Build history of the part. All positions in model axes, mm. A direction names the side the tool comes from. Round coordinates to 2 decimals unless told otherwise and drop trailing zeros. Write each loop counter-clockwise with the first axis right and the second up, starting at its lowest first coordinate (ties: lowest second). Pieces come first, ordered by that corner, then holes. Notation, with made-up numbers: M 82.25,64.25 L 93.25,64.25 A21 ccw 93.25,76.25 Z; hole C -37.5,5.5 d1. An arc over 180 degrees is marked long. Use a Markdown table: item, result.
from build123d import *

# Parameters (mm, degrees)
F0_R     = 3.96875
F1_DEPTH = 6.3246


with BuildPart() as f1:
    # F0 (on Top) → F1 (new body)
    with BuildSketch(Plane.XY):
        with BuildLine():
            Line((61.9125, -152.4), (100.0125, -152.4))
            ThreePointArc((100.0125, -152.4), (108.992756, -148.680256), (112.7125, -139.7))
            Line((112.7125, -139.7), (112.7125, 139.7))
            ThreePointArc((112.7125, 139.7), (108.992756, 148.680256), (100.0125, 152.4))
            Line((100.0125, 152.4), (-100.0125, 152.4))
            ThreePointArc((-100.0125, 152.4), (-108.992756, 148.680256), (-112.7125, 139.7))
            Line((-112.7125, 139.7), (-112.7125, -139.7))
            ThreePointArc((-112.7125, -139.7), (-108.992756, -148.680256), (-100.0125, -152.4))
            Line((-100.0125, -152.4), (-61.9125, -152.4))
            Line((-61.9125, -152.4), (-61.9125, -139.7))
            Line((-61.9125, -139.7), (61.9125, -139.7))
            Line((61.9125, -139.7), (61.9125, -152.4))
        make_face()
        with Locations((-96.8375, -136.525)):
            Circle(F0_R, mode=Mode.SUBTRACT)
        with Locations((96.8375, -136.525)):
            Circle(F0_R, mode=Mode.SUBTRACT)
        with Locations((-80.9625, 139.7)):
            Circle(F0_R, mode=Mode.SUBTRACT)
        with Locations((80.9625, 139.7)):
            Circle(F0_R, mode=Mode.SUBTRACT)
    extrude(amount=F1_DEPTH)


solid = f1.part
Q1. Cut at B-B on x = 42. Give the cut face in (y, z).
Response values:
| item | result |
|---|---|
| outline | M -139.7,0 L 152.4,0 L 152.4,6.32 L -139.7,6.32 Z |
Q2. Drill centre lines: L1, parallel to Y at x = 55, z = 5.25; L2, parallel to Y at x = 96, z = 3; L3, parallel to Y at x = -78.5, z = 2.5. Where is each one in solid material? Low to high.
Response values:
| item | result |
|---|---|
| L1 | y = -139.7 to 152.4 |
| L2 | y = -152.4 to -140.4, -132.65 to 152.4 |
| L3 | y = -152.4 to 136.59, 142.81 to 152.4 |
Q3. Two-plate mould, pull along X, no slides. Class faces 1 (the flat face through (-81, -152.4, 3)), 2 (the flat face through (-112.712, 2, 3)), 3 (the flat face through (61.912, -146, 3)): +X half, -X half, draft (parallel to the pull), parting line (faces both ways), or undercut.
Response values:
| item | result |
|---|---|
| face 1 | draft |
| face 2 | -X half |
| face 3 | undercut |
Q4. Drop flat-ended pins along their axis: P1, Ø1.9, axis at y = -147.5, z = 4, coming from the +X side; P2, Ø5, axis at x = -80.96, y = 139.7, coming from the -Z side; P3, Ø3, axis at y = -148.5, z = 4.5, coming from the -X side. Give the stop position or say it passes through.
Response values:
| item | result |
|---|---|
| P1 | stops at x = 110.71 |
| P2 | passes through |
| P3 | stops at x = -110.4 |
Q5. Which spindle directions (+Z, -Z, +X, -X, +Y, -Y) get a long thin tool onto all of the face, cutting with end or side? Do faces 4 (the flat face through (-61.912, -146, 3)), 5 (the cylindrical face through (108.89, -148.78, 3.12)). Say none if no direction does.
Response values:
| item | result |
|---|---|
| face 4 | +Z, -Z, -Y |
| face 5 | +Z, -Z, +X, -Y |
Q6. Cut at A-A on z = 1.75. Give the cut face in (x, y) (1 decimal), and give its area (3 significant figures).
Response values:
| item | result |
|---|---|
| outline | M -112.7,-139.7 A12.7 ccw -100,-152.4 L -61.9,-152.4 L -61.9,-139.7 L 61.9,-139.7 L 61.9,-152.4 L 100,-152.4 A12.7 ccw 112.7,-139.7 L 112.7,139.7 A12.7 ccw 100,152.4 L -100,152.4 A12.7 ccw -112.7,139.7 Z; hole C -96.8,-136.5 d7.9; hole C -81,139.7 d7.9; hole C 81,139.7 d7.9; hole C 96.8,-136.5 d7.9 |
| area | 66,800 mm2 |
